```python
from build123d import *

# Parameters (mm, degrees)
BOSS_EXTRUDE2_DEPTH     = 4
FILLET1_R               = 4
SKETCH6_R               = 1.5
CUT_EXTRUDE1_DEPTH      = 4
SKETCH3_R               = 1.5
CUT_EXTRUDE2_DEPTH      = 4
SKETCH7_W               = 3.00651588
SKETCH7_H               = 15.442
BOSS_EXTRUDE3_DEPTH     = 35
FILLET2_R               = 3
FILLET3_R               = 3
SKETCH8_W               = 25
SKETCH8_H               = 3
CUT_EXTRUDE6_DEPTH      = 4
CUT_EXTRUDE6_DEPTH_BACK = 4


with BuildPart() as part:
    # Sketch2 → Boss-Extrude2 (new body)
    with BuildSketch(Plane.XY):
        Polygon((-67.081093968, -2.634474623), (-67.081093968, 16.923525377), (-26.695093968, 16.923525377), (-26.695093968, -2.634474623), (-19.075093968, -2.634474623), (-19.075093968, 32.365525377), (-67.081093968, 32.365525377), (-74.701093968, 32.365525377), (-156.39106061, 32.365525377), (-156.39106061, 16.923525377), (-74.701093968, 16.923525377), (-74.701093968, -2.634474623), align=None)
    extrude(amount=BOSS_EXTRUDE2_DEPTH)

    # Fillet1
    fillet1_edges = [part.edges().sort_by_distance(p)[0] for p in [
        (-19.075093968, 32.365525377, 2),
        (-19.075093968, -2.634474623, 2),
        (-74.701093968, -2.634474623, 2),
    ]]
    fillet(fillet1_edges, radius=FILLET1_R)

    # Sketch6 → Cut-Extrude1 (cut)
    with BuildSketch(Plane.XY.offset(4)):
        with Locations((-71.018093968, 12.224525377)):
            Circle(SKETCH6_R)
        with Locations((-22.758093968, 12.224525377)):
            Circle(SKETCH6_R)
        with Locations((-22.758093968, 2.064525377)):
            Circle(SKETCH6_R)
        with Locations((-71.018093968, 2.064525377)):
            Circle(SKETCH6_R)
    extrude(amount=-CUT_EXTRUDE1_DEPTH, mode=Mode.SUBTRACT)

    # Sketch3 → Cut-Extrude2 (cut)
    with BuildSketch(Plane.XY.offset(4)):
        with Locations((-145.701093968, 25.365525377)):
            Circle(SKETCH3_R)
        with Locations((-88.701093968, 25.365525377)):
            Circle(SKETCH3_R)
    extrude(amount=-CUT_EXTRUDE2_DEPTH, mode=Mode.SUBTRACT)

    # Sketch7 → Boss-Extrude3 (add)
    with BuildSketch(Plane.XY.offset(4)):
        with Locations((-154.88780267, 24.644525377)):
            Rectangle(SKETCH7_W, SKETCH7_H)
    extrude(amount=BOSS_EXTRUDE3_DEPTH)

    # Fillet2
    fillet2_edges = [part.edges().sort_by_distance(p)[0] for p in [
        (-153.38454473, 24.644525377, 4),
    ]]
    fillet(fillet2_edges, radius=FILLET2_R)

    # Fillet3
    fillet3_edges = [part.edges().sort_by_distance(p)[0] for p in [
        (-156.39106061, 24.644525377, 0),
    ]]
    fillet(fillet3_edges, radius=FILLET3_R)

    # Sketch8 → Cut-Extrude6 (cut, two sides)
    with BuildSketch(Plane.ZY.offset(156.39106061)) as cut_extrude6_sk:
        with Locations((19.4669967, 24.665525377)):
            Rectangle(SKETCH8_W, SKETCH8_H)
    extrude(amount=CUT_EXTRUDE6_DEPTH, mode=Mode.SUBTRACT)
    extrude(cut_extrude6_sk.sketch, amount=-CUT_EXTRUDE6_DEPTH_BACK, mode=Mode.SUBTRACT)


solid = part.part
```
Source: CAD feature listing. Evaluate the final solid. Frame: model axes, mm. A direction names the side the tool comes from. Round coordinates to 2 decimals unless told otherwise and drop trailing zeros. Loops run counter-clockwise (first coordinate to the right, second up) from the corner with the lowest first, then second, coordinate; pieces in that order, holes last.
(1) Access query for faces 1 (the cylindrical face through (-21.33, 12.68, 2.03)), 2 (the flat face through (-26.695, 7, 2)), 3 (the flat face through (-155, 26.166, 19)), 4 (the flat face through (-74.701, 9, 2)), 5 (the flat face through (-86, 23, 4)). Directions: +Z, -Z, +X, -X, +Y, -Y. A direction counts if a zero-diameter tool reaches every point of the face in a straight line with its end or side. Return the directions, or none.
From the geometry:
face 1: +Z, -Z
face 2: +Z, -Z, -Y
face 3: +X, -X
face 4: +Z, -Z, -X, -Y
face 5: +Z, +X, +Y, -Y
(2) Section query C-C (x = -108). Output: boundary loops of the cut face in (y, z), and give its area (3 significant figures).
From the geometry:
outline: (16.92, 0) - (32.37, 0) - (32.37, 4) - (16.92, 4) - close
area: 61.8 mm2
(3) Section query B-B (y = 20). Output: boundary loops of the cut face in (x, z).
From the geometry:
outline: (-156.39, 3) arc R3 ccw to (-153.39, 0) - (-19.08, 0) - (-19.08, 4) - (-150.38, 4) arc R3 cw to (-153.38, 7) - (-153.38, 39) - (-156.39, 39) - close
(4) Section query A-A (z = 26). Output: boundary loops of the cut face in (x, y), and give its area (3 significant figures).
From the geometry:
outline: (-156.39, 16.92) - (-153.38, 16.92) - (-153.38, 23.17) - (-156.39, 23.17) - close; (-156.39, 26.17) - (-153.38, 26.17) - (-153.38, 32.37) - (-156.39, 32.37) - close
area: 37.4 mm2
(5) Pull-direction query (X, two-part tool) for faces 6 (the cylindrical face through (-155.536, 24.536, 0.902)), 7 (the flat face through (-47, 16.924, 2)), 8 (the flat face through (-19.075, 15, 2)); classes: +X half, -X half, draft (parallel to the pull), parting line (faces both ways), or undercut.
From the geometry:
face 6: -X half
face 7: undercut
face 8: +X half
(6) Contact query for flat-ended pins moving along their axis: pin 1 Ø3 at (y, z) = (5.5, 2.5) entering from -X; pin 2 Ø0.9 at (x, z) = (-155.5, 20) entering from -Y; pin 3 Ø3.5 at (x, y) = (-145.7, 25.37) entering from +Z; pin 4 Ø3.5 at (x, y) = (-88.7, 25.37) entering from -Z. Output: stop coordinate, or through.
From the geometry:
pin 1: stops at x = -74.7
pin 2: stops at y = 16.92
pin 3: stops at z = 4
pin 4: stops at z = 0
(7) Material intervals for probe 1 along X at (y, z) = (16, 2); probe 2 along X at (y, z) = (26.5, 8); probe 3 along Z at (x, y) = (-26.5, 14.5), sorted ascending.
From the geometry:
probe 1: x = -74.7 to -67.08, -26.7 to -19.08
probe 2: x = -156.39 to -153.38
probe 3: z = 0 to 4
